from build123d import *

# Parameters (mm, degrees)
HOLE_WIZARD_M61_D     = 5
HOLE_WIZARD_M61_DEPTH = 27
HOLE_WIZARD_M61_TIP   = 1.502151548


with BuildPart() as part:
    # Эскиз1 → Повернуть1 (revolve)
    with BuildSketch(Plane.XY):
        Polygon((0, 0), (0, 10.65), (-41.861372681, 10.65), (-41.861372681, 10.4), (-54.841568778, 10.4), (-54.841568778, 10), (-66.841568778, 10), (-66.841568778, 0), align=None)
    revolve(axis=Axis((-66.841568778, 0, 0), (1, 0, 0)))

    # Отверстие обработанное метчиком M61
    with Locations(Plane.ZY.offset(66.841568778)):
        with Locations((0, 0)):
            Hole(HOLE_WIZARD_M61_D / 2, depth=HOLE_WIZARD_M61_DEPTH)
            with Locations((0, 0, -(HOLE_WIZARD_M61_DEPTH + HOLE_WIZARD_M61_TIP / 2))):  # 118° drill point
                Cone(0, HOLE_WIZARD_M61_D / 2, HOLE_WIZARD_M61_TIP, mode=Mode.SUBTRACT)

    # Зеркальное отражение1: part across plane


with BuildPart() as part_1:
    add(part.part)
    add(part.part.mirror(Plane.ZY))


solid = part_1.part
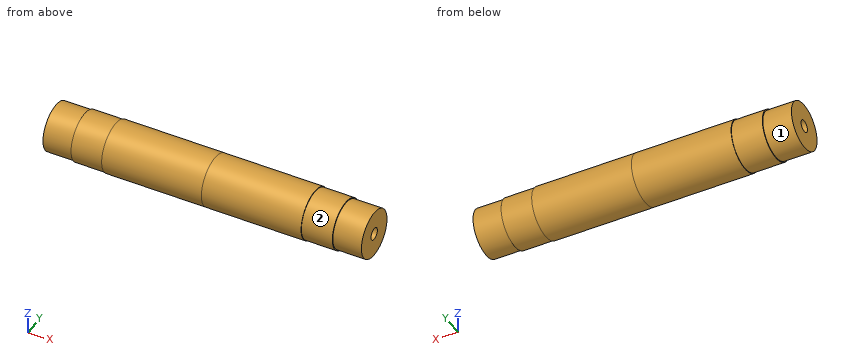
Model file for the job. Use its own axes, mm. Face numbers are marked on the shaded views. A direction names the side the tool comes from. Give positions to 0.01 mm unless a question says otherwise; leave off trailing zeros. Order: outer loops, then holes, each group sorted by start corner. A loop starts at its lowest first (then second) coordinate and runs counter-clockwise, first axis right, second up. Notation, with made-up numbers: M 77.25,40.5 L 126.25,40.5 A34 cw 126.25,71.5 Z; hole C 22.25,9 d9. An arc over 180 degrees is marked long. Put each result on its own line as item: value. Start each with the question number.
(1) Band-saw the part on A-A on z = -6. Give the cut face in (x, y), then the cut area to 3 significant figures.
(2) Band-saw the part on C-C on y = -5.5. Give the cut face in (x, z).
(3) Drill centre lines: L1, parallel to Z at x = -51.25, y = 0; L2, parallel to Z at x = -59.5, y = 0; L3, parallel to Y at x = 42.5, z = 1. Where is each one in solid material? Low to high. Write a range as [from, to].
(4) Pin check, flat tips, straight feed: pin 1 Ø4 at (y, z) = (0, 0) entering from -X; pin 2 Ø1.5 at (x, y) = (-14, 1.5) entering from +Z; pin 3 Ø4.5 at (y, z) = (0, 0) entering from +X. Stop position of each tip, or through.
(5) Tool access for the marked faces 1 and 2: list every direction of +Z, -Z, +X, -X, +Y, -Y with a clear straight run to the whole face (end or side of a thin tool).
(6) Band-saw the part on B-B on x = -26. Give the cut face in (y, z), then the cut area to 3 significant figures.
Results below:
1. outline: M -66.84,-8 L -54.84,-8 L -54.84,-8.49 L -41.86,-8.49 L -41.86,-8.8 L 41.86,-8.8 L 41.86,-8.49 L 54.84,-8.49 L 54.84,-8 L 66.84,-8 L 66.84,8 L 54.84,8 L 54.84,8.49 L 41.86,8.49 L 41.86,8.8 L -41.86,8.8 L -41.86,8.49 L -54.84,8.49 L -54.84,8 L -66.84,8 Z
1. area: 2,300 mm2
2. outline: M -66.84,-8.35 L -54.84,-8.35 L -54.84,-8.83 L -41.86,-8.83 L -41.86,-9.12 L 41.86,-9.12 L 41.86,-8.83 L 54.84,-8.83 L 54.84,-8.35 L 66.84,-8.35 L 66.84,8.35 L 54.84,8.35 L 54.84,8.83 L 41.86,8.83 L 41.86,9.12 L -41.86,9.12 L -41.86,8.83 L -54.84,8.83 L -54.84,8.35 L -66.84,8.35 Z
3. L1: z = [-10.4, -2.5], [2.5, 10.4]
3. L2: z = [-10, -2.5], [2.5, 10]
3. L3: y = [-10.35, -2.29], [2.29, 10.35]
4. pin 1: stops at x = -39.54
4. pin 2: stops at z = 10.62
4. pin 3: stops at x = 39.69
5. face 1: -X
5. face 2: +X
6. outline: C 0,0 d21.3
6. area: 356 mm2
